The model under review builds one solid part; all positions refer to its coordinate system, in mm. Face numbers are marked on the shaded views. A direction names the side the tool comes from. Coordinates: 2 decimals unless noted, no trailing zeros. Order: outer loops, then holes, each group sorted by start corner. A loop starts at its lowest first (then second) coordinate and runs counter-clockwise, first axis right, second up.
```python
from build123d import *

# Parameters (mm, degrees)
SKETCH4_W            = 40
SKETCH4_H            = 80
BOSS_EXTRUDE4_DEPTH  = 5
SKETCH5_W            = 10
SKETCH5_H            = 5
BOSS_EXTRUDE6_DEPTH  = 50
SKETCH7_W            = 10
SKETCH7_H            = 25
SKETCH7_H_2          = 5
BOSS_EXTRUDE7_DEPTH  = 20
SKETCH9_W            = 80
SKETCH9_H            = 5
BOSS_EXTRUDE9_DEPTH  = 10
SKETCH10_W           = 50
SKETCH10_H           = 5
BOSS_EXTRUDE10_DEPTH = 20
SKETCH11_R           = 2.25
CUT_EXTRUDE1_DEPTH   = 25
SKETCH12_R           = 4
SKETCH12_R_2         = 2.25
CUT_EXTRUDE2_DEPTH   = 2
SKETCH15_W           = 5
SKETCH15_H           = 50
BOSS_EXTRUDE11_DEPTH = 20
CUT_EXTRUDE4_REACH   = 89.464
SKETCH16_R           = 2.75
SKETCH19_W           = 5
SKETCH19_H           = 50
BOSS_EXTRUDE12_DEPTH = 5
SKETCH21_W           = 50
SKETCH21_H           = 100
BOSS_EXTRUDE14_DEPTH = 5
SKETCH22_W           = 50
SKETCH22_H           = 10
BOSS_EXTRUDE15_DEPTH = 20
SKETCH24_W           = 35
SKETCH24_H           = 5
CUT_EXTRUDE5_DEPTH   = 50
SKETCH25_W           = 10
SKETCH25_H           = 25
SKETCH25_H_2         = 5
BOSS_EXTRUDE16_DEPTH = 25
SKETCH26_W           = 10
SKETCH26_H           = 5
BOSS_EXTRUDE17_DEPTH = 20
BOSS_EXTRUDE18_START = 2
SKETCH27_R           = 4
SKETCH27_R_2         = 2.25
BOSS_EXTRUDE18_DEPTH = 2
SKETCH28_R           = 2.25
CUT_EXTRUDE6_DEPTH   = 50
SKETCH29_W           = 25
SKETCH29_H           = 5
BOSS_EXTRUDE19_DEPTH = 50
SKETCH31_R           = 2.75
CUT_EXTRUDE7_DEPTH   = 30
SKETCH32_W           = 30
SKETCH32_H           = 45
CUT_EXTRUDE8_DEPTH   = 10
SKETCH33_W           = 30
SKETCH33_H           = 10
CUT_EXTRUDE9_DEPTH   = 30
SKETCH35_R           = 2.1
CUT_EXTRUDE10_DEPTH  = 10


with BuildPart() as part:
    # Sketch4 → Boss-Extrude4 (new body)
    with BuildSketch(Plane(origin=(0, 0, 0), x_dir=(1, 0, 0), z_dir=(0, 1, 0))):
        with Locations((20, 40)):
            Rectangle(SKETCH4_W, SKETCH4_H)
    extrude(amount=BOSS_EXTRUDE4_DEPTH)

    # Sketch5 → Boss-Extrude6 (add)
    with BuildSketch(Plane(origin=(0, 5, 0), x_dir=(1, 0, 0), z_dir=(0, 1, 0))):
        with Locations((35, 52.5)):
            Rectangle(SKETCH5_W, SKETCH5_H)
        with Locations((35, 27.5)):
            Rectangle(SKETCH5_W, SKETCH5_H)
    extrude(amount=BOSS_EXTRUDE6_DEPTH)

    # Sketch7 → Boss-Extrude7 (add)
    with BuildSketch(Plane.XY.offset(-50)):
        with Locations((35, 17.5)):
            Rectangle(SKETCH7_W, SKETCH7_H)
        with Locations((35, 52.5)):
            Rectangle(SKETCH7_W, SKETCH7_H_2)
    extrude(amount=BOSS_EXTRUDE7_DEPTH)

    # Sketch9 → Boss-Extrude9 (add)
    with BuildSketch(Plane.ZY):
        with Locations((-40, 2.5)):
            Rectangle(SKETCH9_W, SKETCH9_H)
    extrude(amount=BOSS_EXTRUDE9_DEPTH)

    # Sketch10 → Boss-Extrude10 (add)
    with BuildSketch(Plane.XY):
        with Locations((15, 2.5)):
            Rectangle(SKETCH10_W, SKETCH10_H)
    extrude(amount=BOSS_EXTRUDE10_DEPTH)

    # Sketch11 → Cut-Extrude1 (cut, symmetric)
    with BuildSketch(Plane.XY.offset(-50)):
        with Locations((35, 40)):
            Circle(SKETCH11_R)
    extrude(amount=CUT_EXTRUDE1_DEPTH, both=True, mode=Mode.SUBTRACT)

    # Sketch12 → Cut-Extrude2 (cut)
    with BuildSketch(Plane.XY.offset(-25)):
        with Locations((35, 40)):
            Circle(SKETCH12_R)
        with Locations((35, 40)):
            Circle(SKETCH12_R_2, mode=Mode.SUBTRACT)
    extrude(amount=-CUT_EXTRUDE2_DEPTH, mode=Mode.SUBTRACT)

    # Sketch15 → Boss-Extrude11 (add)
    with BuildSketch(Plane.ZY.offset(-30)):
        with Locations((-52.5, 30)):
            Rectangle(SKETCH15_W, SKETCH15_H)
        with Locations((-27.5, 30)):
            Rectangle(SKETCH15_W, SKETCH15_H)
    extrude(amount=BOSS_EXTRUDE11_DEPTH)

    # Cut-Extrude4: up to this face of the body (flat: up to its plane)
    cut_extrude4_end = Plane(part.part.faces().sort_by_distance((24.892834991, 29.892834991, -55))[0])
    # Sketch16 → Cut-Extrude4 (cut, up to the picked face)
    with BuildSketch(Plane.XY.offset(-25), mode=Mode.PRIVATE) as cut_extrude4_sk1:
        with Locations((17, 40)):
            Circle(SKETCH16_R)
    cut_extrude4_tool1 = split(extrude(cut_extrude4_sk1.sketch, amount=-CUT_EXTRUDE4_REACH, mode=Mode.PRIVATE), bisect_by=cut_extrude4_end, keep=Keep.BOTH, mode=Mode.PRIVATE)
    add(cut_extrude4_tool1.solids().sort_by(Axis((17, 40, -25), (0, 0, -1)))[0], mode=Mode.SUBTRACT)

    # Sketch19 → Boss-Extrude12 (add)
    with BuildSketch(Plane.ZY.offset(-10)):
        with Locations((-52.5, 30)):
            Rectangle(SKETCH19_W, SKETCH19_H)
        with Locations((-27.5, 30)):
            Rectangle(SKETCH19_W, SKETCH19_H)
    extrude(amount=BOSS_EXTRUDE12_DEPTH)

    # Sketch21 → Boss-Extrude14 (add)
    with BuildSketch(Plane.XZ):
        with Locations((15, -30)):
            Rectangle(SKETCH21_W, SKETCH21_H)
    extrude(amount=BOSS_EXTRUDE14_DEPTH)

    # Sketch22 → Boss-Extrude15 (add)
    with BuildSketch(Plane(origin=(0, 0, -80), x_dir=(-1, 0, 0), z_dir=(0, 0, -1))):
        with Locations((-15, 0)):
            Rectangle(SKETCH22_W, SKETCH22_H)
    extrude(amount=BOSS_EXTRUDE15_DEPTH)

    # Sketch24 → Cut-Extrude5 (cut)
    with BuildSketch(Plane(origin=(0, 55, 0), x_dir=(1, 0, 0), z_dir=(0, 1, 0))):
        with Locations((22.5, 52.5)):
            Rectangle(SKETCH24_W, SKETCH24_H)
    extrude(amount=-CUT_EXTRUDE5_DEPTH, mode=Mode.SUBTRACT)

    # Sketch25 → Boss-Extrude16 (add)
    with BuildSketch(Plane(origin=(0, 0, -50), x_dir=(-1, 0, 0), z_dir=(0, 0, -1))):
        with Locations((-35, 17.5)):
            Rectangle(SKETCH25_W, SKETCH25_H)
        with Locations((-35, 52.5)):
            Rectangle(SKETCH25_W, SKETCH25_H_2)
    extrude(amount=BOSS_EXTRUDE16_DEPTH)

    # Sketch26 → Boss-Extrude17 (add)
    with BuildSketch(Plane(origin=(0, 30, 0), x_dir=(1, 0, 0), z_dir=(0, 1, 0))):
        with Locations((35, 72.5)):
            Rectangle(SKETCH26_W, SKETCH26_H)
    extrude(amount=BOSS_EXTRUDE17_DEPTH)

    # Sketch27 → Boss-Extrude18 (add)
    with BuildSketch(Plane.XY.offset(-27).offset(BOSS_EXTRUDE18_START)):
        with Locations((35, 40)):
            Circle(SKETCH27_R)
        with Locations((35, 40)):
            Circle(SKETCH27_R_2, mode=Mode.SUBTRACT)
    extrude(amount=-BOSS_EXTRUDE18_DEPTH)

    # Sketch28 → Cut-Extrude6 (cut)
    with BuildSketch(Plane.XY.offset(-25)):
        with Locations((35, 40)):
            Circle(SKETCH28_R)
    extrude(amount=-CUT_EXTRUDE6_DEPTH, mode=Mode.SUBTRACT)

    # Sketch29 → Boss-Extrude19 (add)
    with BuildSketch(Plane(origin=(0, 5, 0), x_dir=(1, 0, 0), z_dir=(0, 1, 0))):
        with Locations((17.5, 52.5)):
            Rectangle(SKETCH29_W, SKETCH29_H)
    extrude(amount=BOSS_EXTRUDE19_DEPTH)

    # Sketch31 → Cut-Extrude7 (cut)
    with BuildSketch(Plane.XY.offset(-25)):
        with Locations((17, 40)):
            Circle(SKETCH31_R)
    extrude(amount=-CUT_EXTRUDE7_DEPTH, mode=Mode.SUBTRACT)

    # Sketch32 → Cut-Extrude8 (cut)
    with BuildSketch(Plane(origin=(0, 5, 0), x_dir=(1, 0, 0), z_dir=(0, 1, 0))):
        with Locations((5, 77.5)):
            Rectangle(SKETCH32_W, SKETCH32_H)
        with Locations((5, 2.5)):
            Rectangle(SKETCH32_W, SKETCH32_H)
    extrude(amount=-CUT_EXTRUDE8_DEPTH, mode=Mode.SUBTRACT)

    # Sketch33 → Cut-Extrude9 (cut)
    with BuildSketch(Plane.ZY.offset(10)):
        with Locations((-40, 0)):
            Rectangle(SKETCH33_W, SKETCH33_H)
    extrude(amount=-CUT_EXTRUDE9_DEPTH, mode=Mode.SUBTRACT)

    # Sketch35 → Cut-Extrude10 (cut)
    with BuildSketch(Plane(origin=(0, 5, 0), x_dir=(1, 0, 0), z_dir=(0, 1, 0))):
        with Locations(Location((30, 85, 0), (0, 0, 270))):
            Circle(SKETCH35_R)
        with Locations(Location((30, -5, 0), (0, 0, 270))):
            Circle(SKETCH35_R)
    extrude(amount=-CUT_EXTRUDE10_DEPTH, mode=Mode.SUBTRACT)


solid = part.part
```
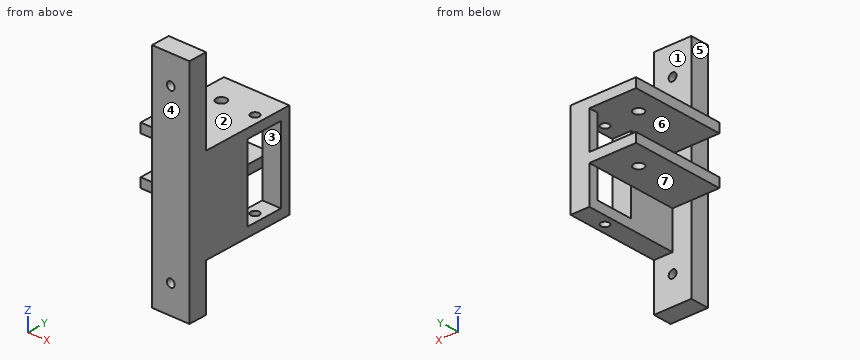
(1) We need section D-D, the plane x = 35. Write out the cut boundary in (y, z), and give its area (4 significant figures).
A:
outline: (-5, -100) - (5, -100) - (5, -75) - (37.75, -75) - (37.75, -70) - (30, -70) - (30, -30) - (37.75, -30) - (37.75, -25) - (5, -25) - (5, 20) - (-5, 20) - close; (42.25, -75) - (55, -75) - (55, -25) - (42.25, -25) - (42.25, -30) - (50, -30) - (50, -70) - (42.25, -70) - close
area: 2,855 mm2
(2) Machinability: for the marked faces 4, 5, 6 and 7, which of the approach directions +Z, -Z, +X, -X, +Y, -Y give a long, thin tool a straight path to every point of the face, cutting with its end or side? Answer none if there is none.
A:
face 4: +Z, -Z, +X, -X, -Y
face 5: +Z, -Z, -X, -Y
face 6: -X
face 7: -Z, -X, +Y
(3) We need section C-C, the plane x = 17. Write out the cut boundary in (y, z).
A:
outline: (5, -55) - (37.25, -55) - (37.25, -50) - (5, -50) - close; (5, -30) - (37.25, -30) - (37.25, -25) - (5, -25) - close; (42.75, -55) - (55, -55) - (55, -50) - (42.75, -50) - close; (42.75, -30) - (55, -30) - (55, -25) - (42.75, -25) - close
(4) Draft analysis for pull direction Y (two halves, no side actions). For the marked faces 1, 2 and 3, state which applies: released by +Y, released by -Y, zero draft, split by the parting line, or undercut.
A:
face 1: released by +Y
face 2: zero draft
face 3: undercut
(5) We need section A-A, the plane z = 5. Write out the cut boundary in (x, y), and give its area (3 significant figures).
A:
outline: (20, -5) - (27.9, -5) - (27.9, 5) - (20, 5) - close; (32.1, -5) - (40, -5) - (40, 5) - (32.1, 5) - close
area: 158 mm2
(6) We need section B-B, the plane y = 32.5. Write out the cut boundary in (x, z).
A:
outline: (5, -55) - (30, -55) - (30, -50) - (5, -50) - close; (5, -30) - (40, -30) - (40, -25) - (5, -25) - close; (30, -75) - (40, -75) - (40, -70) - (30, -70) - close
(7) Wall thickness on probe 1 along Y at (x, z) = (17, -26); probe 2 along Z at (x, y) = (11, 47.5); probe 3 along X at (y, z) = (0.25, 5): over which ranges is each line inside the solid? List them lowest first.
A:
probe 1: y = 5 to 37.25, 42.75 to 55
probe 2: z = -55 to -50, -30 to -25
probe 3: x = 20 to 27.9, 32.1 to 40
(8) For pin 1 Ø1.5 at (y, z) = (52, -36) entering from -X; pin 2 Ø1 at (y, z) = (3.5, 2.5) entering from -X; pin 3 Ø12 at (y, z) = (15.5, -23.5) entering from +X; pin 4 Ø6 at (x, y) = (29, 11) entering from -Z, all flat-tipped, find the tip position at first contact; note any pin that passes through.
A:
pin 1: stops at x = 30
pin 2: stops at x = 20
pin 3: stops at x = 40
pin 4: stops at z = -75
